Verification items for this drawing (mm, ordinates from the low corner). Round coordinates to 2 decimals unless told otherwise and drop trailing zeros. Loops run counter-clockwise (first coordinate to the right, second up) from the corner with the lowest first, then second, coordinate; pieces in that order, holes last. Notation, with made-up numbers: (48, 20) -> (66, 20) arc R12 cw to (66, 38) -> close; hole circle Ø2 at (81, -30). An arc over 180 degrees is marked (long way). One line per item, written item: value. Start each with the question number.
1. Go/stop test with a flat-tipped pin: pin 1 (6 mm diameter, centred on x = 29, y = 9.5, fed in from -Z). Record where the tip stops, or that it passes through.
2. Cross-section at A-A on x = 20. Record the cut outline in (y, z), then the cut area to 3 significant figures.
3. Cross-section at B-B on y = 35. Record the cut outline in (x, z), then the cut area to 3 significant figures.
4. Material ranges on L1, parallel to Y at x = 20, z = 4; L2, parallel to Y at x = 5, z = 3.8; L3, parallel to X at y = 36.5, z = 2.75, recorded low to high.
5. Cross-section at D-D on x = 5. Record the cut outline in (y, z).
6. Release check for a two-part mould opening along X. For the marked faces 1, 2 and 3 record: +X half, -X half, draft (parallel to the pull), parting line (faces both ways), or undercut.
7. Cross-section at C-C on z = 2.7. Count the separate pieces of the cut face and the enclosed holes in it, then the cut area to 3 significant figures.
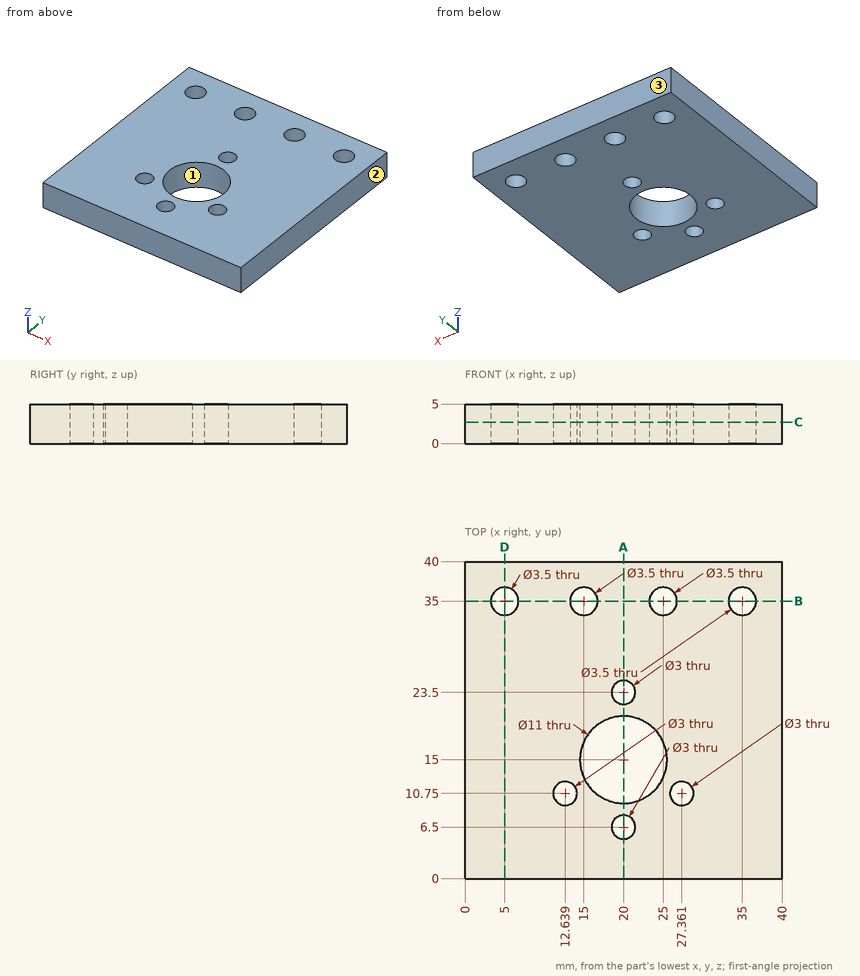
Taken from the geometry:
1. pin 1: stops at z = 0
2. outline: (0, 0) -> (5, 0) -> (5, 5) -> (0, 5) -> close; (8, 0) -> (9.5, 0) -> (9.5, 5) -> (8, 5) -> close; (20.5, 0) -> (22, 0) -> (22, 5) -> (20.5, 5) -> close; (25, 0) -> (40, 0) -> (40, 5) -> (25, 5) -> close
2. area: 115 mm2
3. outline: (0, 0) -> (3.25, 0) -> (3.25, 5) -> (0, 5) -> close; (6.75, 0) -> (13.25, 0) -> (13.25, 5) -> (6.75, 5) -> close; (16.75, 0) -> (23.25, 0) -> (23.25, 5) -> (16.75, 5) -> close; (26.75, 0) -> (33.25, 0) -> (33.25, 5) -> (26.75, 5) -> close; (36.75, 0) -> (40, 0) -> (40, 5) -> (36.75, 5) -> close
3. area: 130 mm2
4. L1: y = 0 to 5, 8 to 9.5, 20.5 to 22, 25 to 40
4. L2: y = 0 to 33.25, 36.75 to 40
4. L3: x = 0 to 4.1, 5.9 to 14.1, 15.9 to 24.1, 25.9 to 34.1, 35.9 to 40
5. outline: (0, 0) -> (33.25, 0) -> (33.25, 5) -> (0, 5) -> close; (36.75, 0) -> (40, 0) -> (40, 5) -> (36.75, 5) -> close
6. face 1: undercut
6. face 2: +X half
6. face 3: draft
7. separate pieces: 1
7. enclosed holes: 9
7. area: 1,440 mm2
